Part model, mm, in its own coordinate system. Round coordinates to 2 decimals unless told otherwise and drop trailing zeros. Loops run counter-clockwise (first coordinate to the right, second up) from the corner with the lowest first, then second, coordinate; pieces in that order, holes last.
Autodesk Inventor part; units mm, degrees
ref_plane "YZ Plane" through (0, 0, 0) normal (1, 0, 0) x (0, 1, 0)
ref_plane "XZ Plane" through (0, 0, 0) normal (0, 1, 0) x (-1, 0, 0)
ref_plane "XY Plane" through (0, 0, 0) normal (0, 0, 1) x (1, 0, 0)
sketch "Sketch1" plane through (0, 0, 0) normal (0, 1, 0) x (-1, 0, 0)
  circle A0 centre (0, 0) radius 6
  dimension "d0" = 12
extrude "Extrusion1" add sketch "Sketch1" along normal blind 150
fillet "Fillet1" radius 5 1 edges at (6, 150, 0)
fillet "Fillet2" radius 5 1 edges at (6, 0, 0)
thread "Thread1"
properties part number "Griff"
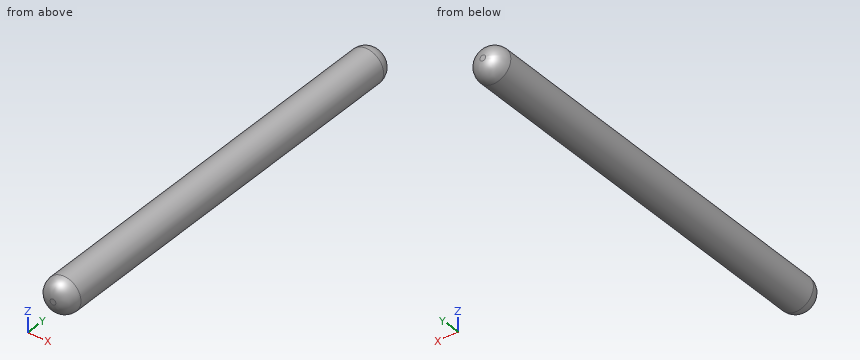
1) Wall check: line 1 along Z through (x, y) = (0.5, 80); line 2 along X through (y, z) = (25, 0.25); line 3 along Y through (x, z) = (-2, 1). Give the ranges that are in metal, low to high.
Values:
line 1: z = -5.98 to 5.98
line 2: x = -5.99 to 5.99
line 3: y = 0.16 to 149.84
2) Drop flat-ended pins along their axis: pin 1 Ø4 at (x, z) = (2, 1) entering from +Y; pin 2 Ø1.5 at (x, z) = (-2.5, 4.5) entering from -Y; pin 3 Ø4 at (y, z) = (52.5, -2.5) entering from +X; pin 4 Ø1 at (x, y) = (3.5, 20.5) entering from +Z. Give the stop position or say it passes through.
Values:
pin 1: stops at y = 150
pin 2: stops at y = 1.33
pin 3: stops at x = 5.98
pin 4: stops at z = 5.2
3) Slice it at A-A, the plane y = 86. Give the cut face in (x, z).
Values:
outline: circle Ø12 at (0, 0)
